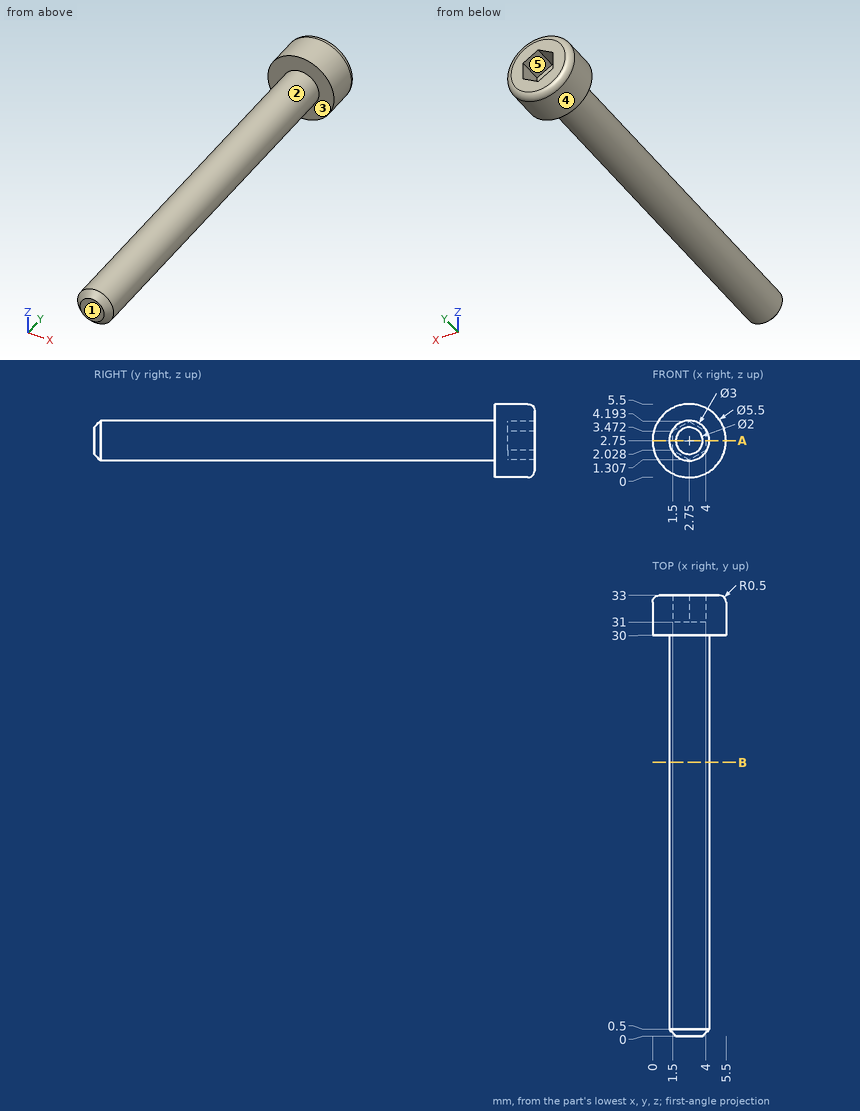
Design review of the part shown in the three views and the two pictorial views. Dimensions are in mm from the part's minimum x, y and z. A direction names the side the tool comes from. Give positions to 0.01 mm unless a question says otherwise; leave off trailing zeros. Loops run counter-clockwise (first coordinate to the right, second up) from the corner with the lowest first, then second, coordinate; pieces in that order, holes last. Notation, with made-up numbers: (-30.5, 63.5) - (28.5, 63.5) arc R35 cw to (28.5, 102.5) - close; hole circle Ø4 at (-7.5, -21.5). An arc over 180 degrees is marked (long way). Use CSV: the item, a comma, the result in double quotes. Start each with the question number.
1. Wall thickness on L1, parallel to Y at x = 3.55, z = 2.8; L2, parallel to Y at x = 2.3, z = 1.05; L3, parallel to Z at x = 1.7, y = 23.5: over which ranges is each line inside the solid? List them lowest first.
2. Add section A-A (z = 2.75). State the section outline as (x, y) points, plus the area to 3 significant figures.
3. Insertion check: P1, Ø1, axis at y = 22.5, z = 0.5, coming from the -X side; P2, Ø1.5, axis at y = 24.5, z = 2.5, coming from the +X side. Each pin has a flat end and moves straight along its axis. Give the tip position at first contact, or say it passes through.
4. Draft analysis for pull direction X (two halves, no side actions). For the marked faces 3, 4 and 5, state which applies: released by +X, released by -X, zero draft, split by the parting line, or undercut.
5. Machinability: for the marked faces 1 and 2, which of the approach directions +Z, -Z, +X, -X, +Y, -Y give a long, thin tool a straight path to every point of the face, cutting with its end or side? Answer none if there is none.
6. Add section B-B (y = 20.5). State the section outline as (x, z) points.
Results found:
1,L1,"y = 0 to 31"
1,L2,"y = 30 to 33"
1,L3,"z = 1.68 to 3.82"
2,outline,"(0, 30) - (1.25, 30) - (1.25, 0.5) - (1.75, 0) - (3.75, 0) - (4.25, 0.5) - (4.25, 30) - (5.5, 30) - (5.5, 32.5) arc R0.5 ccw to (5, 33) - (4, 33) - (4, 31) - (1.5, 31) - (1.5, 33) - (0.5, 33) arc R0.5 ccw to (0, 32.5) - close"
2,area,"101 mm²"
3,P1,"passes through"
3,P2,"stops at x = 4.25"
4,face 3,"zero draft"
4,face 4,"split by the parting line"
4,face 5,"undercut"
5,face 1,"+Z, -Z, +X, -X, -Y"
5,face 2,"-Y"
6,outline,"circle Ø3 at (2.75, 2.75)"
